```python
from build123d import *

# Parameters (mm, degrees)
F0_W     = 50.8
F0_H     = 50.8
F1_DEPTH = 50.8
F2_W     = 38.1
F2_H     = 38.1
F3_DEPTH = 38.1
F4_W     = 50.8
F4_H     = 12.7
F5_DEPTH = 6.35
F6_W     = 25.4
F6_H     = 25.4
F7_DEPTH = 25.4
F8_W     = 6.35
F8_H     = 38.1
F9_DEPTH = 12.7


with BuildPart() as f1:
    # F0 (on Top) → F1 (new body)
    with BuildSketch(Plane.XY):
        with Locations((-25.4, 25.4)):
            Rectangle(F0_W, F0_H)
    extrude(amount=F1_DEPTH)

    # F2 (on face) → F3 (cut)
    with BuildSketch(Plane.XY.offset(50.8)):
        with Locations((-19.05, 19.05)):
            Rectangle(F2_W, F2_H)
    extrude(amount=-F3_DEPTH, mode=Mode.SUBTRACT)

    # F4 (on face) → F5 (join)
    with BuildSketch(Plane.YZ):
        with Locations((25.4, 44.45)):
            Rectangle(F4_W, F4_H)
    extrude(amount=-F5_DEPTH)

    # F6 (on face) → F7 (join)
    with BuildSketch(Plane.YZ):
        with Locations((12.7, 38.1)):
            Rectangle(F6_W, F6_H)
    extrude(amount=-F7_DEPTH)

    # F8 (on face) → F9 (cut)
    with BuildSketch(Plane(origin=(0, 50.8, 0), x_dir=(-1, 0, 0), z_dir=(0, 1, 0))):
        with Locations((9.525, 31.75)):
            Rectangle(F8_W, F8_H)
        with Locations((15.875, 31.75)):
            Rectangle(F8_W, F8_H)
    extrude(amount=-F9_DEPTH, mode=Mode.SUBTRACT)


solid = f1.part
```
Can you work these out from the model? Positions are in its coordinate system, mm. A direction names the side the tool comes from. Coordinates: 2 decimals unless noted, no trailing zeros. Order: outer loops, then holes, each group sorted by start corner. A loop starts at its lowest first (then second) coordinate and runs counter-clockwise, first axis right, second up. Notation, with made-up numbers: (-31.75, 75.25) - (-11.75, 75.25) arc R34 cw to (-11.75, 114.25) - close; hole circle Ø7 at (-37.75, -17). An arc over 180 degrees is marked (long way). Answer in a Markdown table with one row per item.
1. Suppose I cut it at D-D (z = 41). Please give me the cut outline in (x, y).
Reply:
| item | result |
|---|---|
| outline | (-50.8, 0) - (-38.1, 0) - (-38.1, 38.1) - (-19.05, 38.1) - (-19.05, 50.8) - (-50.8, 50.8) - close; (-25.4, 0) - (0, 0) - (0, 50.8) - (-6.35, 50.8) - (-6.35, 25.4) - (-25.4, 25.4) - close |
2. Suppose I cut it at C-C (y = 10.5). Please give me the cut outline in (x, z).
Reply:
| item | result |
|---|---|
| outline | (-50.8, 0) - (0, 0) - (0, 12.7) - (-38.1, 12.7) - (-38.1, 50.8) - (-50.8, 50.8) - close; (-25.4, 25.4) - (0, 25.4) - (0, 50.8) - (-25.4, 50.8) - close |
3. If we mould it in two halves opening along Z, with no side actions, what happens to faces 1 (the flat face through (-3, 32, 38.1)), 2 (the flat face through (-10, 19, 50.8)), 3 (the flat face through (-26, 26, 0))? For each: pulls with the +Z half, pulls with the -Z half, needs draft (parallel to the pull), parting line crosses it, or undercut.
Reply:
| item | result |
|---|---|
| face 1 | undercut |
| face 2 | pulls with the +Z half |
| face 3 | pulls with the -Z half |
4. Suppose I cut it at B-B (z = 31). Please give me the cut outline in (x, y), and give its area (3 significant figures).
Reply:
| item | result |
|---|---|
| outline | (-50.8, 0) - (-38.1, 0) - (-38.1, 38.1) - (-19.05, 38.1) - (-19.05, 50.8) - (-50.8, 50.8) - close; (-25.4, 0) - (0, 0) - (0, 25.4) - (-25.4, 25.4) - close; (-6.35, 38.1) - (0, 38.1) - (0, 50.8) - (-6.35, 50.8) - close |
| area | 1,610 mm^2 |
5. For pin 1 (12 mm diameter, centred on x = -14, y = 27.5, fed in from +Z); pin 2 (1.9 mm diameter, centred on x = -4, z = 24, fed in from -Y), each with a flat end and sliding along its axis, tell me the tip position at first contact or that it passes through.
Reply:
| item | result |
|---|---|
| pin 1 | stops at z = 50.8 |
| pin 2 | stops at y = 38.1 |
6. If I drill on line 1 along Z through (x, y) = (-5, 14); line 2 along X through (y, z) = (39, 26); line 3 along X through (y, z) = (22, 32.5), over which ranges is the centre line in solid material (lowest first)?
Reply:
| item | result |
|---|---|
| line 1 | z = 0 to 12.7, 25.4 to 50.8 |
| line 2 | x = -50.8 to -19.05, -6.35 to 0 |
| line 3 | x = -50.8 to -38.1, -25.4 to 0 |
7. Suppose I cut it at A-A (x = -9). Please give me the cut outline in (y, z).
Reply:
| item | result |
|---|---|
| outline | (0, 0) - (50.8, 0) - (50.8, 12.7) - (0, 12.7) - close; (0, 25.4) - (25.4, 25.4) - (25.4, 50.8) - (0, 50.8) - close |
8. For faces 4 (the flat face through (-29, 38.1, 32)), 5 (the flat face through (-19.05, 45, 31)), 6 (the flat face through (-25.4, 13, 38)), which set-ups out of +Z, -Z, +X, -X, +Y, -Y let a thin tool reach every point of the face, with its end or its side?
Reply:
| item | result |
|---|---|
| face 4 | +Z |
| face 5 | +Z, +Y |
| face 6 | +Z, -Y |
